```python
from build123d import *

# Parameters (mm, degrees)
F0_R     = 50
F0_R_2   = 40
F0_R_3   = 28.75
F1_DEPTH = 5
F2_DEPTH = 10
F3_W     = 62
F3_H     = 62
F3_R     = 28.75
F4_DEPTH = 3


with BuildPart() as f1:
    # F0 (on Top) → F1 (new body)
    with BuildSketch(Plane.XY):
        Circle(F0_R)
        Circle(F0_R_2, mode=Mode.SUBTRACT)
        Circle(F0_R_2)
        Circle(F0_R_3, mode=Mode.SUBTRACT)
    extrude(amount=F1_DEPTH)

    # F0 (on Top) → F2 (join)
    with BuildSketch(Plane.XY):
        Circle(F0_R_2)
        Circle(F0_R_3, mode=Mode.SUBTRACT)
    extrude(amount=F2_DEPTH)

    # F3 (on face) → F4 (cut)
    with BuildSketch(Plane(origin=(0, 0, 0), x_dir=(1, 0, 0), z_dir=(0, 0, -1))):
        Rectangle(F3_W, F3_H)
        Circle(F3_R, mode=Mode.SUBTRACT)
    extrude(amount=-F4_DEPTH, mode=Mode.SUBTRACT)


solid = f1.part
```
Can you work these out from the model? Positions are in its coordinate system, mm. A direction names the side the tool comes from. Round coordinates to 2 decimals unless told otherwise and drop trailing zeros. Loops run counter-clockwise (first coordinate to the right, second up) from the corner with the lowest first, then second, coordinate; pieces in that order, holes last.
Item 1: If we mould it in two halves opening along Y, with no side actions, what happens to faces 4 (the cylindrical face through (-8.67, -39.05, 7.46)), 5 (the flat face through (26, -17, 10)), 6 (the flat face through (-21, 21, 3))? For each: +Y half, -Y half, draft (parallel to the pull), parting line (faces both ways), or undercut.
Item 2: Which directions (+Z, -Z, +X, -X, +Y, -Y) give clear straight access to the entire face, cutting with the end or side of a thin tool? Please do faces 1 (the flat face through (-22, 34, 5)), 2 (the cylindrical face through (-6.232, -28.066, 6.451)), 3 (the flat face through (31, 0, 1)).
Item 3: Suppose I cut it at C-C, the plane z = 7.5. Write out the boundary of the cut face in (x, y), then the cut area to 3 significant figures.
Item 4: Please list where these lines run through material, in increasing order: L1, parallel to Y at x = 0, z = 6; L2, parallel to Z at x = 30.5, y = -26.
Item 5: Suppose I cut it at D-D, the plane y = 32.5. Write out the boundary of the cut face in (x, z).
Item 6: Will these pins go through, and if not, where does the flat tip stop? pin 1 Ø0.9 at (y, z) = (-13.5, 1.5) entering from +X; pin 2 Ø3 at (x, y) = (-31, -31) entering from +Z; pin 3 Ø2.5 at (y, z) = (8, 1) entering from -X.
Item 7: Suppose I cut it at A-A, the plane y = 0. Write out the boundary of the cut face in (x, z), then the cut area to 4 significant figures.
Reported:
1. face 4: parting line
1. face 5: draft
1. face 6: undercut
2. face 1: +Z
2. face 2: +Z, -Z
2. face 3: -Z
3. outline: circle Ø80 at (0, 0); hole circle Ø57.5 at (0, 0)
3. area: 2,430 mm2
4. L1: y = -40 to -28.75, 28.75 to 40
4. L2: z = 3 to 5
5. outline: (-38, 0) - (38, 0) - (38, 5) - (23.32, 5) - (23.32, 10) - (-23.32, 10) - (-23.32, 5) - (-38, 5) - close
6. pin 1: stops at x = 48.27
6. pin 2: stops at z = 5
6. pin 3: stops at x = -49.54
7. outline: (-50, 0) - (-31, 0) - (-31, 3) - (-28.75, 3) - (-28.75, 10) - (-40, 10) - (-40, 5) - (-50, 5) - close; (28.75, 3) - (31, 3) - (31, 0) - (50, 0) - (50, 5) - (40, 5) - (40, 10) - (28.75, 10) - close
7. area: 311.5 mm2
